from build123d import *

# Parameters (mm, degrees)
BOSS_EXTRUDE1_DEPTH      = 70
SKETCH2_W                = 23
SKETCH2_H                = 17
BOSS_EXTRUDE2_DEPTH      = 2
SKETCH3_W                = 23
SKETCH3_H                = 17
BOSS_EXTRUDE3_DEPTH      = 2
SKETCH4_W                = 23
SKETCH4_H                = 17
BOSS_EXTRUDE4_DEPTH      = 1
BOSS_EXTRUDE4_DEPTH_BACK = 1
SKETCH6_R                = 0.5
CUT_EXTRUDE7_DEPTH       = 57
SKETCH7_R                = 0.5
CUT_EXTRUDE8_DEPTH       = 57


with BuildPart() as part:
    # Sketch1 → Boss-Extrude1 (new body)
    with BuildSketch(Plane.XY):
        Polygon((-11.5, 8.5), (-11.5, -8.5), (11.5, -8.5), (11.5, 8.5), (9.5, 8.5), (9.5, 7), (9.5, -7), (-9.5, -7), (-9.5, 7), (-9.5, 8.5), align=None)
    extrude(amount=BOSS_EXTRUDE1_DEPTH)

    # Sketch2 → Boss-Extrude2 (add)
    with BuildSketch(Plane.XY.offset(70)):
        Rectangle(SKETCH2_W, SKETCH2_H)
    extrude(amount=-BOSS_EXTRUDE2_DEPTH)

    # Sketch3 → Boss-Extrude3 (add)
    with BuildSketch(Plane(origin=(0, 0, 0), x_dir=(-1, 0, 0), z_dir=(0, 0, -1))):
        Rectangle(SKETCH3_W, SKETCH3_H)
    extrude(amount=-BOSS_EXTRUDE3_DEPTH)

    # Sketch4 → Boss-Extrude4 (add, two sides)
    with BuildSketch(Plane(origin=(0, 0, 35), x_dir=(-1, 0, 0), z_dir=(0, 0, -1))) as boss_extrude4_sk:
        Rectangle(SKETCH4_W, SKETCH4_H)
    extrude(amount=BOSS_EXTRUDE4_DEPTH)
    extrude(boss_extrude4_sk.sketch, amount=-BOSS_EXTRUDE4_DEPTH_BACK)

    # Sketch6 → Cut-Extrude7 (cut)
    with BuildSketch(Plane(origin=(11.5, 0, 0), x_dir=(0, 0, -1), z_dir=(1, 0, 0))):
        with Locations((-35, -4)):
            Circle(SKETCH6_R)
    cut_extrude7 = extrude(amount=-CUT_EXTRUDE7_DEPTH, mode=Mode.SUBTRACT)

    # Sketch7 → Cut-Extrude8 (cut)
    with BuildSketch(Plane(origin=(11.5, 0, 0), x_dir=(0, 0, -1), z_dir=(1, 0, 0))):
        with Locations((-52.5, -4)):
            Circle(SKETCH7_R)
    cut_extrude8 = extrude(amount=-CUT_EXTRUDE8_DEPTH, mode=Mode.SUBTRACT)

    # Mirror1: Cut-Extrude8 across plane
    add(cut_extrude8.mirror(Plane(origin=(0, 0, 35), x_dir=(1, 0, 0), z_dir=(0, 0, -1))), mode=Mode.SUBTRACT)

    # Mirror2: Cut-Extrude7 across plane
    add(cut_extrude7.mirror(Plane.ZX), mode=Mode.SUBTRACT)


solid = part.part
CAD build for the part. Positions are in the model's coordinates, mm. A direction names the side the tool comes from. Give positions to 0.01 mm unless a question says otherwise; leave off trailing zeros. Loops run counter-clockwise (first coordinate to the right, second up) from the corner with the lowest first, then second, coordinate; pieces in that order, holes last. Notation, with made-up numbers: M 81,83.5 L 134,83.5 A33 cw 134,122.5 Z; hole C 69,62.5 d11. An arc over 180 degrees is marked long. Answer in a Markdown table with one row per item. Add a question column.
Item 1: Mould opens along Z. For faces 1 (the face through (-9.5, 1, 18)), 2 (the face through (0, 0, 70)), 3 (the face through (0, 0, 0)) say: +Z half, -Z half, draft (parallel to the pull), parting line (faces both ways), or undercut.
Item 2: Tool access for faces 4 (the face through (11.5, 0, 35)), 5 (the face through (9.5, 1, 52)): list every direction of +Z, -Z, +X, -X, +Y, -Y with a clear straight run to the whole face (end or side of a thin tool).
Item 3: Band-saw the part on B-B on y = -1.25. Give the cut face in (x, z), then the cut area to 3 significant figures.
Item 4: Band-saw the part on A-A on x = -8. Give the cut face in (y, z).
Item 5: Drop a flat-ended pin along its axis: P1, Ø1, axis at x = 0.5, z = 13, coming from the +Y side. Give the stop position or say it passes through.
Item 6: Probe probe 1 along Y at (x, z) = (-4.25, 35); probe 2 along Z at (x, y) = (5, 2.25); probe 3 along X at (y, z) = (0, 63.5). List the from-to ranges inside material, lowest first.
Item 7: Band-saw the part on C-C on z = 12. Give the cut face in (x, y).
Reply:
| question | item | result |
|---|---|---|
| 1 | face 1 | undercut |
| 1 | face 2 | +Z half |
| 1 | face 3 | -Z half |
| 2 | face 4 | +Z, -Z, +X, +Y, -Y |
| 2 | face 5 | +Y |
| 3 | outline | M -11.5,0 L 11.5,0 L 11.5,70 L -11.5,70 Z; hole M -9.5,2 L 9.5,2 L 9.5,34 L -9.5,34 Z; hole M -9.5,36 L 9.5,36 L 9.5,68 L -9.5,68 Z |
| 3 | area | 394 mm^2 |
| 4 | outline | M -8.5,0 L 8.5,0 L 8.5,2 L -7,2 L -7,34 L 8.5,34 L 8.5,36 L -7,36 L -7,68 L 8.5,68 L 8.5,70 L -8.5,70 Z; hole C -4,35 d1; hole C 4,35 d1 |
| 5 | P1 | stops at y = -7 |
| 6 | probe 1 | y = -8.5 to -4.5, -3.5 to 3.5, 4.5 to 8.5 |
| 6 | probe 2 | z = 0 to 2, 34 to 36, 68 to 70 |
| 6 | probe 3 | x = -11.5 to -9.5, 9.5 to 11.5 |
| 7 | outline | M -11.5,-8.5 L 11.5,-8.5 L 11.5,8.5 L 9.5,8.5 L 9.5,-7 L -9.5,-7 L -9.5,8.5 L -11.5,8.5 Z |
